Source: CAD feature listing. Evaluate the final solid. Frame: model axes, mm. Face numbers are marked on the shaded views. A direction names the side the tool comes from. Give positions to 0.01 mm unless a question says otherwise; leave off trailing zeros. Write each loop counter-clockwise with the first axis right and the second up, starting at its lowest first coordinate (ties: lowest second). Pieces come first, ordered by that corner, then holes. Notation, with made-up numbers: (51, 77) - (91, 77) arc R24 ccw to (91, 101) - close; hole circle Ø6 at (79.5, 37.25). An arc over 180 degrees is marked (long way). Answer as a JSON object with one key per item and string values. Group by question number.
from build123d import *

# Parameters (mm, degrees)
F0_W           = 15.6
F0_H           = 11.5
F1_DEPTH       = 5.4
F2_W           = 15.6
F2_H           = 3
F3_DEPTH       = 0.4
F6_D           = 2
F6_DEPTH       = 5
F6_TIP         = 0.600860619
F6_ON_F5_D     = 2
F6_ON_F5_DEPTH = 5
F6_ON_F5_TIP   = 0.600860619
F8_DEPTH       = 25
F10_DEPTH      = 3
F12_D          = 4


with BuildPart() as f1:
    # F0 (on Front) → F1 (new body)
    with BuildSketch(Plane.XZ):
        with Locations((0, -1.15)):
            Rectangle(F0_W, F0_H)
    extrude(amount=-F1_DEPTH)

    # F2 (on face) → F3 (join)
    with BuildSketch(Plane.XZ):
        with Locations((0, -5.4)):
            Rectangle(F2_W, F2_H)
    extrude(amount=F3_DEPTH)

    # F6
    with Locations(Plane.YZ.offset(7.8)):
        with Locations((2.9, -1.9)):
            Hole(F6_D / 2, depth=F6_DEPTH)
            with Locations((0, 0, -(F6_DEPTH + F6_TIP / 2))):  # 118° drill point
                Cone(0, F6_D / 2, F6_TIP, mode=Mode.SUBTRACT)

    # F6 on F5
    with Locations(Plane(origin=(-7.8, 0, 0), x_dir=(0, -1, 0), z_dir=(-1, 0, 0))):
        with Locations((-2.9, -1.9)):
            Hole(F6_ON_F5_D / 2, depth=F6_ON_F5_DEPTH)
            with Locations((0, 0, -(F6_ON_F5_DEPTH + F6_ON_F5_TIP / 2))):  # 118° drill point
                Cone(0, F6_ON_F5_D / 2, F6_ON_F5_TIP, mode=Mode.SUBTRACT)

    # F7 (on face) → F8 (cut)
    with BuildSketch(Plane(origin=(0, 0, -6.9), x_dir=(1, 0, 0), z_dir=(0, 0, -1))):
        Polygon((-6.3, -2.9), (-7.8, -1.4), (-7.8, -4.4), align=None)
        Polygon((7.8, -4.4), (7.8, -1.4), (6.3, -2.9), align=None)
    extrude(amount=-F8_DEPTH, mode=Mode.SUBTRACT)

    # F9 (on face) → F10 (cut, through all)
    with BuildSketch(Plane(origin=(0, 0, -6.9), x_dir=(1, 0, 0), z_dir=(0, 0, -1))):
        Polygon((-0.25, 0.4), (0, 0.15), (0.25, 0.4), align=None)
    extrude(amount=-F10_DEPTH, mode=Mode.SUBTRACT)

    # F12 (through all)
    with Locations(Plane.XZ):
        with Locations((-4, 2.1), (4, 2.1)):
            Hole(F12_D / 2)


solid = f1.part
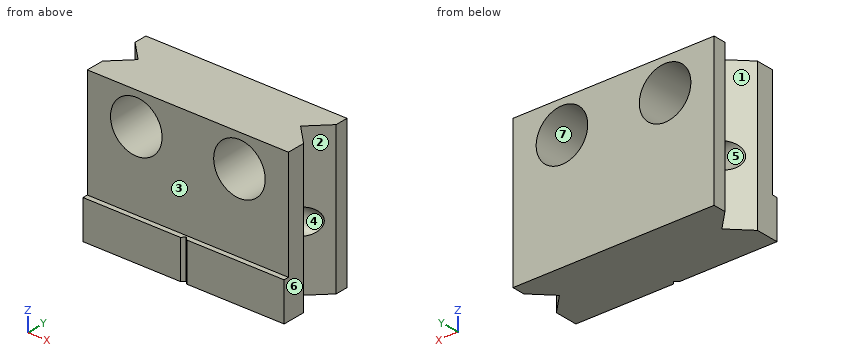
Q1. Reachability of the marked faces 1, 2, 3 and 4 from +Z, -Z, +X, -X, +Y, -Y: full face, straight path, thin tool, end or side. Return the list, or none.
Q2. Section A-A on x = -4. Return the cut outline in (y, z), then the cut area to 3 significant figures.
Q3. First-contact query: pin 1 Ø3.5 at (x, z) = (-4, 2.1) entering from -Y; pin 2 Ø2.5 at (y, z) = (2.9, -1.9) entering from +X; pin 3 Ø2.5 at (y, z) = (2.9, -1.9) entering from -X. Flat tips, straight axial feed; report the tip coordinate or a pass-through.
Q4. Section C-C on y = 0.5. Return the cut outline in (x, z).
Q5. Draft query along X for the marked faces 5, 6 and 7. Return one class per face: released by +X, released by -X, zero draft, split by the parting line, or undercut.
Q6. Section D-D on z = -5. Return the cut outline in (x, y).
Q7. Section B-B on z = 2.1. Return the cut outline in (x, y).
Q8. Ray query, probe 1 along Y at (x, z) = (4.6, -1.9); probe 2 along Z at (x, y) = (4.25, 3.8); probe 3 along X at (y, z) = (3.15, 3). Return the intervals inside material, ascending. Write a range as [from, to].
Taken from the geometry:
{
 "1": {"face 1": "+Z, -Z, -X", "face 2": "+Z, -Z, +X", "face 3": "+Z, +X, -X, -Y", "face 4": "+X"},
 "2": {"outline": "(-0.4, -6.9) - (5.4, -6.9) - (5.4, 0.1) - (0, 0.1) - (0, -3.9) - (-0.4, -3.9) - close; (0, 4.1) - (5.4, 4.1) - (5.4, 4.6) - (0, 4.6) - close; hole circle Ø2 at (2.9, -1.9)", "area": "38.6 mm²"},
 "3": {"pin 1": "passes through", "pin 2": "stops at x = 7.55", "pin 3": "stops at x = -7.55"},
 "4": {"outline": "(-7.8, -6.9) - (7.8, -6.9) - (7.8, 4.6) - (-7.8, 4.6) - close; hole circle Ø4 at (-4, 2.1); hole circle Ø4 at (4, 2.1)"},
 "5": {"face 5": "zero draft", "face 6": "released by +X", "face 7": "undercut"},
 "6": {"outline": "(-7.8, -0.4) - (-0.25, -0.4) - (0, -0.15) - (0.25, -0.4) - (7.8, -0.4) - (7.8, 1.4) - (6.3, 2.9) - (7.8, 4.4) - (7.8, 5.4) - (-7.8, 5.4) - (-7.8, 4.4) - (-6.3, 2.9) - (-7.8, 1.4) - close"},
 "7": {"outline": "(-7.8, 0) - (-6, 0) - (-6, 5.4) - (-7.8, 5.4) - (-7.8, 4.4) - (-6.3, 2.9) - (-7.8, 1.4) - close; (-2, 0) - (2, 0) - (2, 5.4) - (-2, 5.4) - close; (6, 0) - (7.8, 0) - (7.8, 1.4) - (6.3, 2.9) - (7.8, 4.4) - (7.8, 5.4) - (6, 5.4) - close"},
 "8": {"probe 1": "y = [0, 1.9], [3.9, 5.4]", "probe 2": "z = [-6.9, -2.34], [-1.46, 0.12], [4.08, 4.6]", "probe 3": "x = [-6.55, -5.79], [-2.21, 2.21], [5.79, 6.55]"}
}
